Can you work these out from the drawing? Everything is in mm from the part's minimum corner. A direction names the side the tool comes from. Give positions to 0.01 mm unless a question says otherwise; leave off trailing zeros. Order: outer loops, then holes, each group sorted by start corner. A loop starts at its lowest first (then second) coordinate and runs counter-clockwise, first axis right, second up. Notation, with made-up numbers: (85, 17) - (104, 17) arc R28 cw to (104, 56) - close; hole circle Ø9 at (25, 26). An arc over 180 degrees is marked (long way). Answer as a JSON object with one key per item and string values.
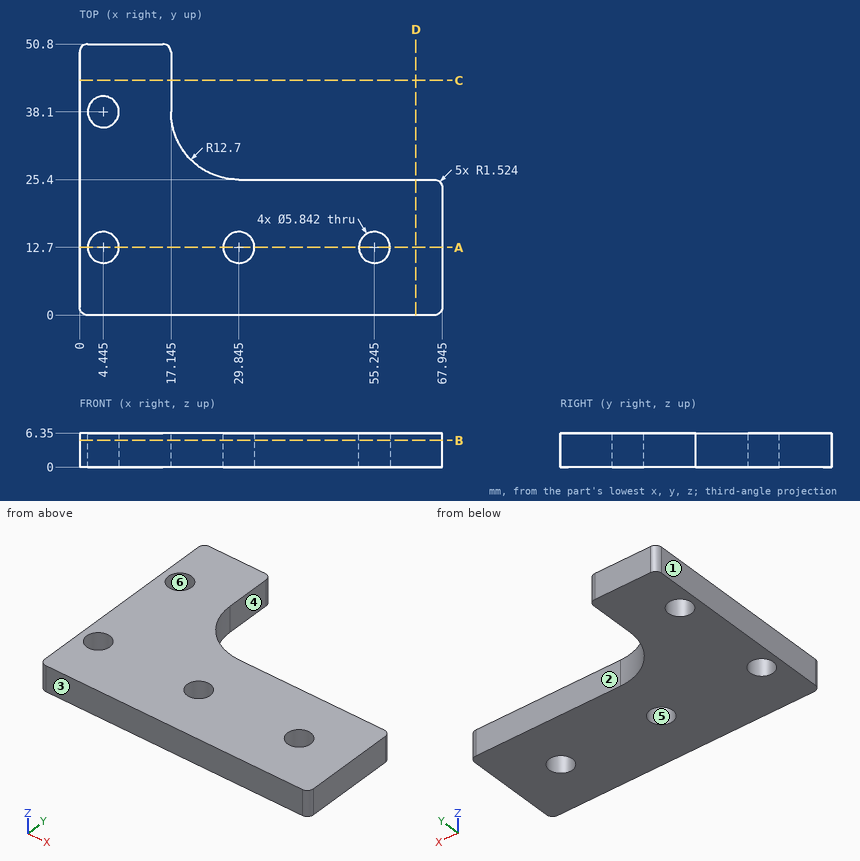
Q1. I'm going to push flat-ended pins straight in: pin 1 Ø7.5 at (x, y) = (29.845, 12.7) entering from -Z; pin 2 Ø5.5 at (x, y) = (4.445, 12.7) entering from -Z; pin 3 Ø1.9 at (x, z) = (48.5, 4.5) entering from +Y. Where does each tip first touch, or does it pass through?
Recorded:
{"pin 1": "stops at z = 0", "pin 2": "passes through", "pin 3": "stops at y = 25.4"}
Q2. If we section it at A-A, the plane y = 12.7: Please give me the cut outline in (x, z) (3 decimals).
Recorded:
{"outline": "(0, 0) - (1.524, 0) - (1.524, 6.35) - (0, 6.35) - close; (7.366, 0) - (26.924, 0) - (26.924, 6.35) - (7.366, 6.35) - close; (32.766, 0) - (52.324, 0) - (52.324, 6.35) - (32.766, 6.35) - close; (58.166, 0) - (67.945, 0) - (67.945, 6.35) - (58.166, 6.35) - close"}
Q3. If we section it at B-B, the plane z = 5: Please give me the cut outline in (x, y) (3 decimals).
Recorded:
{"outline": "(0, 1.524) arc R1.524 ccw to (1.524, 0) - (66.421, 0) arc R1.524 ccw to (67.945, 1.524) - (67.945, 23.876) arc R1.524 ccw to (66.421, 25.4) - (29.845, 25.4) arc R12.7 cw to (17.145, 38.1) - (17.145, 49.276) arc R1.524 ccw to (15.621, 50.8) - (1.524, 50.8) arc R1.524 ccw to (0, 49.276) - close; hole circle Ø5.842 at (4.445, 12.7); hole circle Ø5.842 at (4.445, 38.1); hole circle Ø5.842 at (29.845, 12.7); hole circle Ø5.842 at (55.245, 12.7)"}
Q4. I need wall thicknesses on L1, parallel to X at y = 38, z = 2.75; L2, parallel to Y at x = 3, z = 4.5; L3, parallel to Y at x = 61, z = 1. Which ranges of each line are inside material? Lowest first, please.
Recorded:
{"L1": "x = 0 to 1.53, 7.36 to 17.15", "L2": "y = 0 to 10.16, 15.24 to 35.56, 40.64 to 50.8", "L3": "y = 0 to 25.4"}
Q5. Which directions (+Z, -Z, +X, -X, +Y, -Y) give clear straight access to the entire face, cutting with the end or side of a thin tool? Please do the marked faces 1 and 2.
Recorded:
{"face 1": "+Z, -Z, -X, +Y, -Y", "face 2": "+Z, -Z, +X, +Y"}
Q6. If we section it at D-D, the plane x = 63: Please give me the cut outline in (y, z).
Recorded:
{"outline": "(0, 0) - (25.4, 0) - (25.4, 6.35) - (0, 6.35) - close"}
Q7. We'd pull the mould along Y, two halves only. Please class the marked faces 3, 4, 5 and 6: released by +Y, released by -Y, zero draft, split by the parting line, or undercut.
Recorded:
{"face 3": "released by -Y", "face 4": "zero draft", "face 5": "undercut", "face 6": "undercut"}
Q8. If we section it at C-C, the plane y = 44: Please give me the cut outline in (x, z) (3 decimals), then the cut area to 3 significant figures.
Recorded:
{"outline": "(0, 0) - (17.145, 0) - (17.145, 6.35) - (0, 6.35) - close", "area": "109 mm^2"}
